Part model, mm, in its own coordinate system. A direction names the side the tool comes from. Give positions to 0.01 mm unless a question says otherwise; leave off trailing zeros. Use CSV: the item, a comma, the result in double quotes. Start each with the question number.
1. Drop flat-ended pins along their axis: pin 1 Ø5 at (x, z) = (9.5, 193.5) entering from -Y; pin 2 Ø1.5 at (y, z) = (10, 60) entering from -X; pin 3 Ø2.5 at (x, z) = (9.5, 222) entering from -Y. Give the stop position or say it passes through.
2. Drill centre lines: line 1 along Y through (x, z) = (10, 86); line 2 along Y through (x, z) = (3.75, 213); line 3 along Y through (x, z) = (13.5, 319). Where is each one in solid material? Low to high. Write a range as from..to.
3. 3-axis set-ups, long thin cutter, end or side, ignore diameter. For faces 1 (the face through (10, 6.1, 177)), 2 (the face through (6.1, 10, 177)), 3 (the face through (10, 13.9, 177)), 4 (the face through (0, 16, 177)): which of +Z, -Z, +X, -X, +Y, -Y reach the whole face in a straight line?
4. Mould opens along Y. For faces 5 (the face through (20, 16, 177)), 6 (the face through (16, 20, 177)), 7 (the face through (13.9, 10, 177)) say: pulls with the +Y half, pulls with the -Y half, needs draft (parallel to the pull), parting line crosses it, or undercut.
from build123d import *

# Parameters (mm, degrees)
SKETCH1_R           = 2.5
BOSS_EXTRUDE1_DEPTH = 360
FILLET1_R           = 1
FILLET2_R           = 0.5
FILLET3_R           = 0.5
FILLET4_R           = 0.5
FILLET5_R           = 0.5


with BuildPart() as part:
    # Sketch1 → Boss-Extrude1 (new body)
    with BuildSketch(Plane.XY):
        Polygon((13.2, 0), (13.2, 1.8), (15.45, 1.8), (15.45, 3.6), (12.95, 6.1), (7.05, 6.1), (4.55, 3.6), (4.55, 1.8), (6.8, 1.8), (6.8, 0), (0, 0), (0, 6.8), (1.8, 6.8), (1.8, 4.55), (3.6, 4.55), (6.1, 7.05), (6.1, 12.95), (3.6, 15.45), (1.8, 15.45), (1.8, 13.2), (0, 13.2), (0, 20), (6.8, 20), (6.8, 18.2), (4.55, 18.2), (4.55, 16.4), (7.05, 13.9), (12.95, 13.9), (15.45, 16.4), (15.45, 18.2), (13.2, 18.2), (13.2, 20), (20, 20), (20, 13.2), (18.2, 13.2), (18.2, 15.45), (16.4, 15.45), (13.9, 12.95), (13.9, 7.05), (16.4, 4.55), (18.2, 4.55), (18.2, 6.8), (20, 6.8), (20, 0), align=None)
        with Locations((10, 10)):
            Circle(SKETCH1_R, mode=Mode.SUBTRACT)
    extrude(amount=BOSS_EXTRUDE1_DEPTH)

    # Fillet1
    fillet1_edges = [part.edges().sort_by_distance(p)[0] for p in [
        (0, 0, 180),
        (0, 20, 180),
        (20, 20, 180),
        (20, 0, 180),
    ]]
    fillet(fillet1_edges, radius=FILLET1_R)

    # Fillet2
    fillet2_edges = [part.edges().sort_by_distance(p)[0] for p in [
        (4.55, 18.2, 180),
        (4.55, 16.4, 180),
        (7.05, 13.9, 180),
        (12.95, 13.9, 180),
        (15.45, 16.4, 180),
        (15.45, 18.2, 180),
    ]]
    fillet(fillet2_edges, radius=FILLET2_R)

    # Fillet3
    fillet3_edges = [part.edges().sort_by_distance(p)[0] for p in [
        (18.2, 15.45, 180),
        (16.4, 15.45, 180),
        (13.9, 12.95, 180),
        (13.9, 7.05, 180),
        (16.4, 4.55, 180),
        (18.2, 4.55, 180),
    ]]
    fillet(fillet3_edges, radius=FILLET3_R)

    # Fillet4
    fillet4_edges = [part.edges().sort_by_distance(p)[0] for p in [
        (1.8, 4.55, 180),
        (3.6, 4.55, 180),
        (6.1, 7.05, 180),
        (6.1, 12.95, 180),
        (3.6, 15.45, 180),
        (1.8, 15.45, 180),
    ]]
    fillet(fillet4_edges, radius=FILLET4_R)

    # Fillet5
    fillet5_edges = [part.edges().sort_by_distance(p)[0] for p in [
        (15.45, 1.8, 180),
        (15.45, 3.6, 180),
        (12.95, 6.1, 180),
        (7.05, 6.1, 180),
        (4.55, 3.6, 180),
        (4.55, 1.8, 180),
    ]]
    fillet(fillet5_edges, radius=FILLET5_R)


solid = part.part
Output:
1,pin 1,"stops at y = 6.03"
1,pin 2,"stops at x = 6.1"
1,pin 3,"stops at y = 6.1"
2,line 1,"y = 6.1..7.5, 12.5..13.9"
2,line 2,"y = 0..4.7, 15.3..20"
2,line 3,"y = 0..1.8, 5.55..14.45, 18.2..20"
3,face 1,"+Z, -Z, -Y"
3,face 2,"+Z, -Z, -X"
3,face 3,"+Z, -Z, +Y"
3,face 4,"+Z, -Z, -X, +Y, -Y"
4,face 5,"needs draft"
4,face 6,"pulls with the +Y half"
4,face 7,"undercut"
